Read the model definition and answer for the solid it produces. Units are mm, in the model's axes. A direction names the side the tool comes from. Give positions to 0.01 mm unless a question says otherwise; leave off trailing zeros. Loops run counter-clockwise (first coordinate to the right, second up) from the corner with the lowest first, then second, coordinate; pieces in that order, holes last. Notation, with made-up numbers: (20, 24) - (74, 24) arc R11 cw to (74, 39) - close; hole circle Ø8 at (51, 70). An arc over 180 degrees is marked (long way). Write item = value, one per line. Start each with the question number.
Autodesk Inventor part; units mm, degrees
ref_plane "Work Plane2" through (0, 3.2, 0) normal (0, 1, 0) x (-1, 0, 0)
ref_plane "Work Plane4" through (0, 5, 0) normal (0, 1, 0) x (-1, 0, 0)
ref_plane "YZ Plane" through (0, 0, 0) normal (1, 0, 0) x (0, 1, 0)
sketch "Sketch1" plane through (0, 0, 0) normal (0, 0, 1) x (1, 0, 0)
  circle A0 centre (0, 0) radius 3.2
  dimension "d0" = 6.4
extrude "Extrusion1" add sketch "Sketch1" along normal blind 90
ref_plane "Work Plane2" through (0, 3.2, 0) normal (0, 1, 0) x (-1, 0, 0)
sketch "Sketch7" plane through (0, 3.2, 0) normal (0, 1, 0) x (-1, 0, 0)
  line L0 (2.5, 50) -> (-2.5, 50)
  line L1 (-2.5, 50) -> (-2.5, 45)
  line L2 (-2.5, 45) -> (2.5, 45)
  line L3 (2.5, 45) -> (2.5, 50)
  line L4 (-3.2, 0) -> (3.2, 0)
  line L5 (3.2, 90) -> (-3.2, 90)
  point P0 (0, 0)
  dimension "d30" = 5
  dimension "d31" = 5
  dimension "d32" = 2.5
  dimension "d42" = 40
extrude "Extrusion6" add sketch "Sketch7" against normal blind 9.4 and the other way blind 3
sketch "Sketch9" plane through (0, 0, 0) normal (0, 0, -1) x (-1, 0, 0)
  circle A0 centre (0, 0) radius 5
  dimension "d43" = 10
extrude "Extrusion8" add sketch "Sketch9" along normal blind 10
sketch "Sketch10" plane through (0, 0, -10) normal (0, 0, -1) x (-1, 0, 0)
  arc A0 (-2.8284, 1) -> (2.8284, 1) centre (0, 0) ccw
  line L0 (-2.8284, 1) -> (2.8284, 1)
  dimension "d46" = 6
  dimension "d47" = 1
extrude "Extrusion9" cut sketch "Sketch10" against normal blind 7
ref_plane "Work Plane4" through (0, 5, 0) normal (0, 1, 0) x (-1, 0, 0)
sketch "Sketch12" plane through (0, 5, 0) normal (0, 1, 0) x (-1, 0, 0)
  circle A0 centre (0, -6.5) radius 0.8
  line L0 (-5, -10) -> (5, -10)
  point P0 (0, 0)
  dimension "d54" = 1.6
  dimension "d55" = 3.5
extrude "Extrusion11" cut sketch "Sketch12" against normal up to next
properties part number "Rotation"
1. For a pull along X with two mould halves and no side action, classify faces 1 (the cylindrical face through (-2.539, 1.947, 44.37)), 2 (the flat face through (0, 5, 50)), 3 (the cylindrical face through (0, -3, -7)) as released by +X, released by -X, zero draft, split by the parting line, or undercut.
2. Given P1, Ø2, axis at y = -4, z = 47, coming from the -X side; P2, Ø4, axis at y = 3.5, z = 9, coming from the +X side; P3, Ø3.5, axis at y = 3, z = 47.5, coming from the -X side, each flat-ended and moving along its own axis, determine where each tip first touches the part or whether it passes through.
3. A cutting plane is placed at A-A on z = 48. Give the vertices of the cut face in (x, y).
4. A cutting plane is placed at B-B on y = 0. Give the vertices of the cut face in (x, z).
5. A tool of negligible diameter and unlimited length cuts with its end or side. For faces 4 (the flat face through (0, -1, -3)), 5 (the flat face through (2.5, -4, 48)), 6 (the flat face through (-3.3, -1, 0)), 7 (the flat face through (2.5, 4, 48)), from which of +Z, -Z, +X, -X, +Y, -Y can it reach the whole face along a straight path? Write none if from no direction.
6. A cutting plane is placed at C-C on z = 28. Give the vertices of the cut face in (x, y), and give its area (3 significant figures).
7. Consider line 1 along Z through (x, y) = (0, 4.1); line 2 along Y through (x, z) = (-2.5, 83); line 3 along X through (y, z) = (2, 44). Determine where each line is inside the solid, lowest interval first. Write a range as [from, to].
Reply:
q1.face_1 = split by the parting line
q1.face_2 = zero draft
q1.face_3 = undercut
q2.P1 = -2.5
q2.P2 = 2.83
q2.P3 = -2.95
q3.outline = (-2.5, -6.2) - (2.5, -6.2) - (2.5, -2) arc R3.2 ccw to (2.5, 2) - (2.5, 6.2) - (-2.5, 6.2) - (-2.5, 2) arc R3.2 ccw to (-2.5, -2) - close
q4.outline = (-5, -10) - (-3, -10) - (-3, -3) - (3, -3) - (3, -10) - (5, -10) - (5, 0) - (3.2, 0) - (3.2, 90) - (-3.2, 90) - (-3.2, 0) - (-5, 0) - close
q5.face_4 = -Z
q5.face_5 = +Z, +X, -Y
q5.face_6 = none
q5.face_7 = +Z, +X, +Y
q6.outline = circle Ø6.4 at (0, 0)
q6.area = 32.2 mm^2
q7.line_1 = [-10, -7.3], [-5.7, 0], [45, 50]
q7.line_2 = [-2, 2]
q7.line_3 = [-2.5, 2.5]
